The listing builds one solid part. Answer for the finished solid, in the listing's coordinates (mm). Face numbers are marked on the shaded views. A direction names the side the tool comes from. Coordinates: 2 decimals unless noted, no trailing zeros. Order: outer loops, then holes, each group sorted by start corner. A loop starts at its lowest first (then second) coordinate and runs counter-clockwise, first axis right, second up. Notation, with made-up numbers: (56, 89.25) -> (79, 89.25) arc R18 cw to (79, 105.25) -> close; hole circle Ø11 at (37.25, 10). An arc over 180 degrees is marked (long way). Return JSON: item names as keys, results as strings.
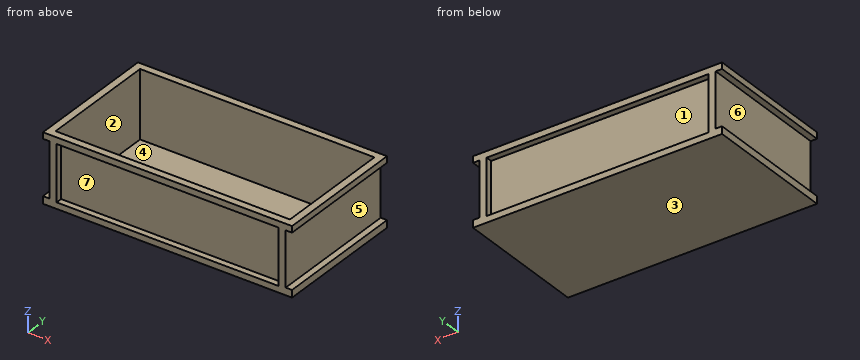
```python
from build123d import *

# Parameters (mm, degrees)
SKETCH_W          = 1186
SKETCH_H          = 632
PAD_DEPTH         = 326
SKETCH001_W       = 30
SKETCH001_H       = 261
POCKET_DEPTH      = 3081.716821
POCKET_DEPTH_BACK = 3081.716821
SKETCH002_W       = 1056
SKETCH002_H       = 266
POCKET001_DEPTH   = 30
SKETCH003_W       = 1116
SKETCH003_H       = 562
POCKET002_DEPTH   = 321.001


with BuildPart() as part:
    # Sketch → Pad (new body)
    with BuildSketch(Plane.XY):
        Rectangle(SKETCH_W, SKETCH_H)
    extrude(amount=PAD_DEPTH)

    # Sketch001 → Pocket (cut, two sides)
    with BuildSketch(Plane.XZ) as pocket_sk:
        with Locations((578, 165.5)):
            Rectangle(SKETCH001_W, SKETCH001_H)
    pocket = extrude(amount=-POCKET_DEPTH, mode=Mode.SUBTRACT) + extrude(pocket_sk.sketch, amount=POCKET_DEPTH_BACK, mode=Mode.SUBTRACT)

    # Mirrored: Pocket across Sketch001 V_Axis
    add(pocket.mirror(Plane(origin=(0, 0, 0), x_dir=(0, -1, 0), z_dir=(1, 0, 0))), mode=Mode.SUBTRACT)

    # Sketch002 → Pocket001 (cut)
    with BuildSketch(Plane.XZ.offset(286)):
        with Locations((0, 163)):
            Rectangle(SKETCH002_W, SKETCH002_H)
    pocket001 = extrude(amount=POCKET001_DEPTH, mode=Mode.SUBTRACT)

    # Mirrored001: Pocket001 across XZ
    add(pocket001.mirror(Plane.XZ), mode=Mode.SUBTRACT)

    # Sketch003 → Pocket002 (cut, through all)
    with BuildSketch(Plane.XY.offset(5)):
        Rectangle(SKETCH003_W, SKETCH003_H)
    extrude(amount=POCKET002_DEPTH, mode=Mode.SUBTRACT)


solid = part.part
```
Item 1: The part is cut by section C-C on x = 1.5. Determine the outline of the cut face in (y, z), plus the area to 3 significant figures.
Answer list:
{"outline": "(-316, 0) -> (316, 0) -> (316, 30) -> (286, 30) -> (286, 296) -> (316, 296) -> (316, 326) -> (281, 326) -> (281, 5) -> (-281, 5) -> (-281, 326) -> (-316, 326) -> (-316, 296) -> (-286, 296) -> (-286, 30) -> (-316, 30) -> close", "area": "9,670 mm2"}
Item 2: Which of the six approach directions +Z, -Z, +X, -X, +Y, -Y give full straight-line access (tool end or side, diameter ignored) to the marked faces 4, 5, 6 and 7?
Answer list:
{"face 4": "+Z", "face 5": "+X, +Y, -Y", "face 6": "-X, +Y, -Y", "face 7": "-Y"}
Item 3: The part is cut by section A-A on z = 265. Determine the outline of the cut face in (x, y).
Answer list:
{"outline": "(-563, -316) -> (-528, -316) -> (-528, -286) -> (528, -286) -> (528, -316) -> (563, -316) -> (563, 316) -> (528, 316) -> (528, 286) -> (-528, 286) -> (-528, 316) -> (-563, 316) -> close; hole (-558, -281) -> (558, -281) -> (558, 281) -> (-558, 281) -> close"}
Item 4: Flat-ended cylindrical pins translate along their axes: pin 1 (15 mm diameter, centred on x = 578.5, y = -112, fed in from -Z); pin 2 (12 mm diameter, centred on y = 163, z = 98.5, fed in from +X); pin 3 (3 mm diameter, centred on x = -204.5, y = 22, fed in from +Z); pin 4 (4 mm diameter, centred on x = 355.5, z = 47, fed in from +Y). Find the tip coordinate at first contact, or state that the pin passes through.
Answer list:
{"pin 1": "z = 0", "pin 2": "x = 563", "pin 3": "z = 5", "pin 4": "y = 286"}
Item 5: Determine the mould class of the marked faces 1, 2 and 3 for opening direction Y: pulls with the +Y half, pulls with the -Y half, needs draft (parallel to the pull), parting line crosses it, or undercut.
Answer list:
{"face 1": "pulls with the +Y half", "face 2": "undercut", "face 3": "needs draft"}
Item 6: The part is cut by section B-B on y = -99. Determine the outline of the cut face in (x, z).
Answer list:
{"outline": "(-593, 0) -> (593, 0) -> (593, 35) -> (563, 35) -> (563, 296) -> (593, 296) -> (593, 326) -> (558, 326) -> (558, 5) -> (-558, 5) -> (-558, 326) -> (-593, 326) -> (-593, 296) -> (-563, 296) -> (-563, 35) -> (-593, 35) -> close"}
Item 7: Find the intervals of material crossed by probe 1 along X at (y, z) = (12.5, 24); probe 2 along Y at (x, z) = (47, 103.5); probe 3 along X at (y, z) = (-25, 281.5), in increasing order.
Answer list:
{"probe 1": "-593 to -558, 558 to 593", "probe 2": "-286 to -281, 281 to 286", "probe 3": "-563 to -558, 558 to 563"}
